```python
from build123d import *

# Parameters (mm, degrees)
F0_W      = 63.5
F0_H      = 36.0719883448
F1_DEPTH  = 25.4
F2_DEPTH  = 62.992
F4_W      = 47.7636682294
F4_H      = 23.5122792056
F5_DEPTH  = 34.29
F3_W      = 47.4535489879
F3_H      = 23.8223956531
F6_DEPTH  = 34.29
F8_DEPTH  = 25.4
F9_DEPTH  = 25.4
F11_DEPTH = 41.402


with BuildPart() as f1:
    # F0 (on Front) → F1 (new body)
    with BuildSketch(Plane.XZ):
        with Locations((-40.8926705517, 18.0359941724)):
            Rectangle(F0_W, F0_H)
    extrude(amount=F1_DEPTH)

    # F2 (add): a face of the model
    f2_faces = [f1.faces().sort_by_distance(p)[0] for p in [
        (-40.8926705517, 0, 18.0359941724),
    ]]
    extrude(f2_faces, amount=F2_DEPTH)

    # F4 (on face) → F5 (cut)
    with BuildSketch(Plane.XZ.offset(25.4)):
        with Locations((-33.0245046664, 24.315848742)):
            Rectangle(F4_W, F4_H)
    extrude(amount=-F5_DEPTH, mode=Mode.SUBTRACT)

    # F3 (on face) → F6 (cut)
    with BuildSketch(Plane(origin=(0, 62.992, 0), x_dir=(-1, 0, 0), z_dir=(0, 1, 0))):
        with Locations((32.8694450457, 24.1607905182)):
            Rectangle(F3_W, F3_H)
    extrude(amount=-F6_DEPTH, mode=Mode.SUBTRACT)

    # F8 (cut): a face of the model
    f8_faces = [f1.faces().sort_by_distance(p)[0] for p in [
        (-9.1426705517, 18.6122366805, 11.6054298815),
    ]]
    extrude(f8_faces, amount=-F8_DEPTH, mode=Mode.SUBTRACT)

    # F7 (on face) → F9 (cut)
    with BuildSketch(Plane.YZ.offset(-56.5962195396)):
        Polygon((62.992, 36.0719883448), (45.847, 36.0719883448), (62.992, 12.2495926917), align=None)
    extrude(amount=-F9_DEPTH, mode=Mode.SUBTRACT)

    # F10 (on face) → F11 (cut)
    with BuildSketch(Plane.XZ.offset(-8.89)):
        Polygon((-34.5426705517, 36.0719883448), (-56.9063387811, 36.0719883448), (-34.5426705517, 12.5597091392), align=None)
    extrude(amount=-F11_DEPTH, mode=Mode.SUBTRACT)


solid = f1.part
```
Input: part model. Units: mm. Frame: model coordinates. A direction names the side the tool comes from. Round coordinates to 2 decimals unless told otherwise and drop trailing zeros. Loops run counter-clockwise (first coordinate to the right, second up) from the corner with the lowest first, then second, coordinate; pieces in that order, holes last.
1) Pin query (flat end, axial travel): pin 1 (11 mm diameter, centred on x = -50, y = 51.5, fed in from +Z); pin 2 (5 mm diameter, centred on y = 27, z = 24, fed in from +X); pin 3 (7 mm diameter, centred on y = -0.5, z = 28.5, fed in from +X); pin 4 (8 mm diameter, centred on x = -59, y = 23.5, fed in from -Z). Return the tip coordinate at first contact, or that it passes through.
Ans:
pin 1: stops at z = 12.25
pin 2: stops at x = -43.05
pin 3: stops at x = -56.91
pin 4: stops at z = 0
2) Section query C-C on z = 23. Return the cut outline in (x, y), plus the area to 3 significant figures.
Ans:
outline: (-72.64, -25.4) - (-56.91, -25.4) - (-56.91, 8.89) - (-44.47, 8.89) - (-44.47, 28.7) - (-56.6, 28.7) - (-56.6, 55.25) - (-72.64, 55.25) - close
area: 1,520 mm2
3) Set-up query: faces 1 (the flat face through (-50, 28.702, 19)), 2 (the flat face through (-34.543, 18, 6)), 3 (the flat face through (-51, 8.89, 19)). Return all of +Z, -Z, +X, -X, +Y, -Y with unobstructed straight access to the full face (end or side cutting, diameter ignored); none if empty.
Ans:
face 1: +Z, +X, +Y
face 2: +Z, -Z, +X, +Y, -Y
face 3: +Z, +X, -Y
4) Material intervals for line 1 (X direction, y = -7, z = 24); line 2 (Y direction, x = -53, z = 17); line 3 (X direction, y = 40, z = 22), sorted ascending.
Ans:
line 1: x = -72.64 to -56.91
line 2: y = 8.89 to 28.7
line 3: x = -72.64 to -56.6
5) Section query B-B on x = -61.5. Return the cut outline in (y, z).
Ans:
outline: (-25.4, 0) - (62.99, 0) - (62.99, 12.25) - (45.85, 36.07) - (-25.4, 36.07) - close
6) Section query D-D on x = -45. Return the cut outline in (y, z), plus the area to 3 significant figures.
Ans:
outline: (-25.4, 0) - (62.99, 0) - (62.99, 12.25) - (28.7, 12.25) - (28.7, 23.55) - (8.89, 23.55) - (8.89, 12.56) - (-25.4, 12.56) - close
area: 1,320 mm2
7) Section query A-A on y = 37.5. Return the cut outline in (x, z), plus the area to 3 significant figures.
Ans:
outline: (-72.64, 0) - (-34.54, 0) - (-34.54, 12.25) - (-56.6, 12.25) - (-56.6, 35.75) - (-56.91, 36.07) - (-72.64, 36.07) - close
area: 849 mm2
